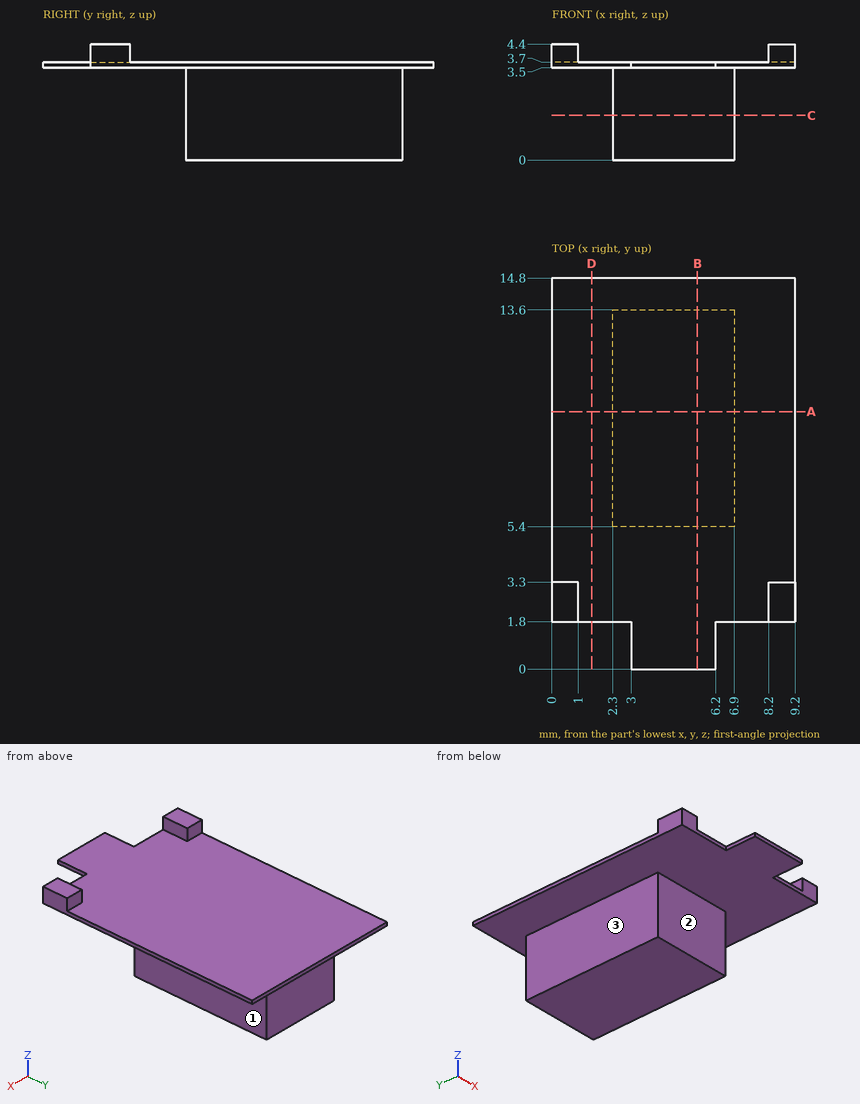
Drawing for the job (mm, zero at the part's lowest x, y, z). A direction names the side the tool comes from. Give positions to 0.01 mm unless a question says otherwise; leave off trailing zeros. Write each loop counter-clockwise with the first axis right and the second up, starting at its lowest first coordinate (ties: lowest second). Pieces come first, ordered by that corner, then holes. Notation, with made-up numbers: M 41.25,10 L 63.25,10 A17 cw 63.25,35 Z; hole C -7,88.5 d8. An arc over 180 degrees is marked long. Use CSV: the item, a comma, the result in double quotes.
Item 1: Slice it at A-A on y = 9.75. Write the cut outline in (x, z).
Taken from the geometry:
outline,"M 0,3.5 L 2.3,3.5 L 2.3,0 L 6.9,0 L 6.9,3.5 L 9.2,3.5 L 9.2,3.7 L 0,3.7 Z"
Item 2: Which spindle directions (+Z, -Z, +X, -X, +Y, -Y) get a long thin tool onto all of the face, cutting with end or side? Do the marked faces 1, 2 and 3. Say none if no direction does.
Taken from the geometry:
face 1,"-Z, +X, +Y, -Y"
face 2,"-Z, +X, -X, -Y"
face 3,"-Z, -X, +Y, -Y"
Item 3: Slice it at C-C on z = 1.7. Write the cut outline in (x, y), plus the area to 3 significant figures.
Taken from the geometry:
outline,"M 2.3,5.4 L 6.9,5.4 L 6.9,13.6 L 2.3,13.6 Z"
area,"37.7 mm²"
Item 4: Pin check, flat tips, straight feed: P1, Ø1, axis at x = 7, z = 4, coming from the -Y side; P2, Ø2, axis at y = 3.5, z = 2, coming from the -X side; P3, Ø1, axis at x = 5, z = 2, coming from the +Y side; P4, Ø1.5, axis at x = 1.5, y = 11.5, coming from the +Z side. Stop position of each tip, or through.
Taken from the geometry:
P1,"stops at y = 1.8"
P2,"passes through"
P3,"stops at y = 13.6"
P4,"stops at z = 3.7"
Item 5: Drill centre lines: probe 1 along Y at (x, z) = (2.5, 0.4); probe 2 along Z at (x, y) = (0.5, 6.25); probe 3 along Z at (x, y) = (5.5, 13.25). Where is each one in solid material? Low to high.
Taken from the geometry:
probe 1,"y = 5.4 to 13.6"
probe 2,"z = 3.5 to 3.7"
probe 3,"z = 0 to 3.7"
Item 6: Slice it at D-D on x = 1.5. Write the cut outline in (y, z), plus the area to 3 significant figures.
Taken from the geometry:
outline,"M 1.8,3.5 L 14.8,3.5 L 14.8,3.7 L 1.8,3.7 Z"
area,"2.60 mm²"
Item 7: Slice it at B-B on x = 5.5. Write the cut outline in (y, z).
Taken from the geometry:
outline,"M 0,3.5 L 5.4,3.5 L 5.4,0 L 13.6,0 L 13.6,3.5 L 14.8,3.5 L 14.8,3.7 L 0,3.7 Z"
